The figure shows three views and two pictorial views of one solid part (mm, origin at its lowest corner). Answer the questions. Coordinates: 2 decimals unless noted, no trailing zeros. Loops run counter-clockwise (first coordinate to the right, second up) from the corner with the lowest first, then second, coordinate; pieces in that order, holes last. Notation, with made-up numbers: (24, 3.5) - (36, 3.5) arc R28 ccw to (36, 37.5) - close; hole circle Ø3 at (-19, 6.5). An arc over 180 degrees is marked (long way). Return JSON: item names as keys, results as strings. Group by question number.
1. Section B-B (z = 23.5) is taken. Write down the section's boundary in (x, y) (1 decimal).
2. Section A-A (x = 0.7) is taken. Write down the section's boundary in (y, z) (1 decimal), and give its area (3 significant figures).
3. Section C-C (y = 35) is taken. Write down the section's boundary in (x, z).
4. Find the intervals of material crossed by line 1 along Y through (x, z) = (0.1, 17); line 2 along Y through (x, z) = (0.85, 4.5); line 3 along Z through (x, y) = (0.55, 31) (1 decimal), in increasing order.
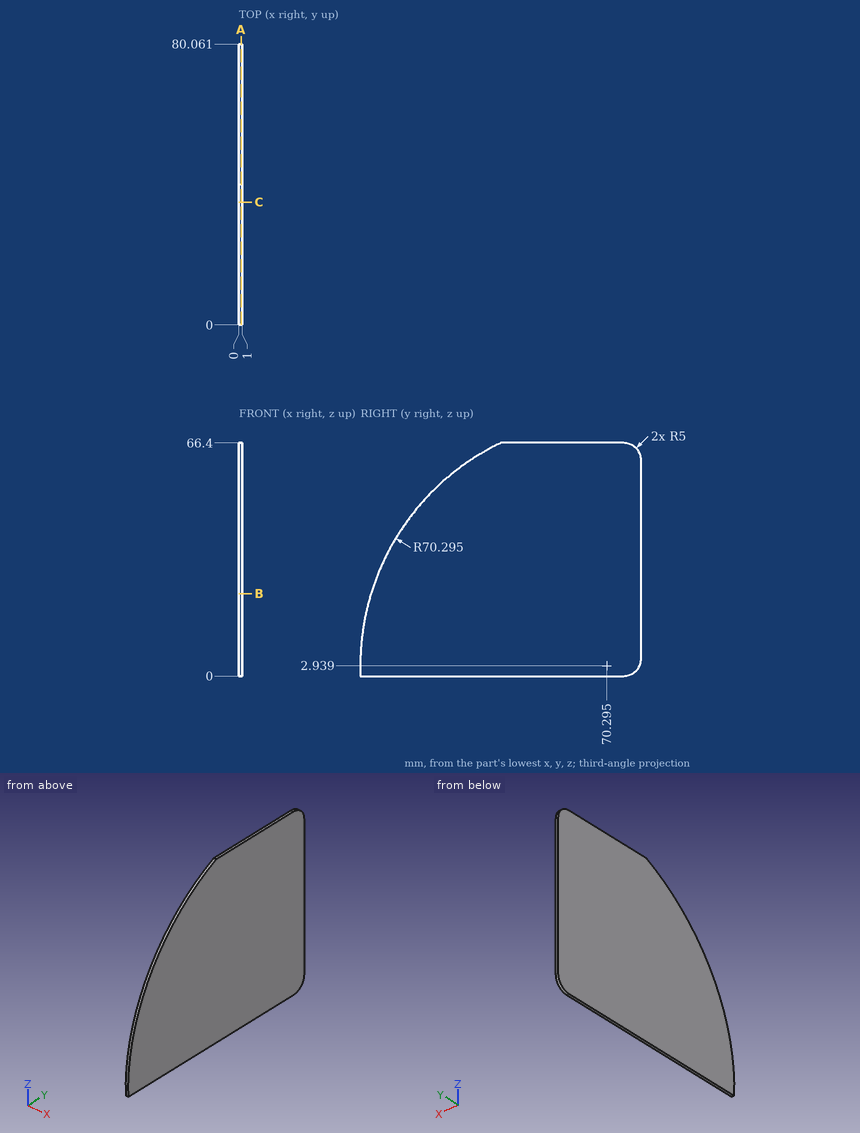
The answers:
{
 "1": {"outline": "(0, 3.1) - (1, 3.1) - (1, 80.1) - (0, 80.1) - close"},
 "2": {"outline": "(0.1, 0) - (75.1, 0) arc R5 ccw to (80.1, 5) - (80.1, 61.4) arc R5 ccw to (75.1, 66.4) - (40.1, 66.4) arc R70.3 ccw to start", "area": "4,590 mm2"},
 "3": {"outline": "(0, 0) - (1, 0) - (1, 63.73) - (0, 63.73) - close"},
 "4": {"line 1": "y = 1.42 to 80.06", "line 2": "y = 0.02 to 80.04", "line 3": "z = 0 to 61.2"}
}
